Work out the finished part from the listing and answer in its coordinate system (mm). Face numbers are marked on the shaded views. Coordinates: 2 decimals unless noted, no trailing zeros. Order: outer loops, then holes, each group sorted by start corner. A loop starts at its lowest first (then second) coordinate and runs counter-clockwise, first axis right, second up. Notation, with made-up numbers: (-20, 19.5) -> (4, 19.5) arc R18 cw to (4, 54.5) -> close; hole circle Ø11 at (55, 88). An arc over 180 degrees is marked (long way). Use one line per item in the form item = value.
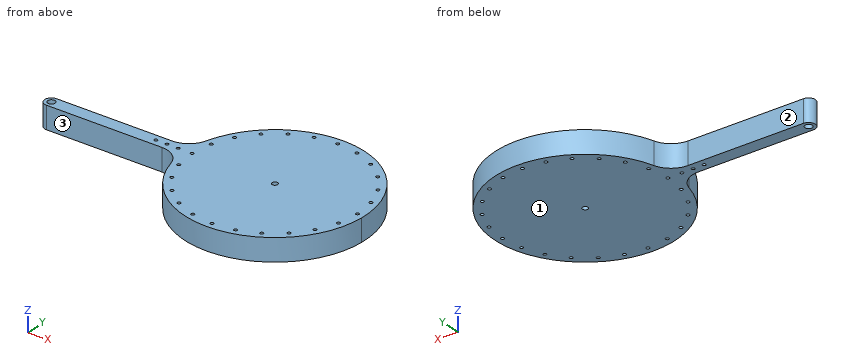
from build123d import *

# Parameters (mm, degrees)
SKETCH1_R           = 1.45
SKETCH1_R_2         = 1.450000001
SKETCH1_R_3         = 3.250000001
SKETCH1_R_4         = 2.5
BOSS_EXTRUDE2_DEPTH = 20


with BuildPart() as part:
    # Sketch1 → Boss-Extrude2 (new body)
    with BuildSketch(Plane.XY):
        with BuildLine():
            Line((-155.352886895, 10.211716756), (-51.913748531, 10.211716756))
            ThreePointArc((-51.913748531, 10.211716756), (-39.74822347, 6.086224622), (-32.601576204, -4.588283244))
            ThreePointArc((-32.601576204, -4.588283244), (53.610301025, -63.284580406), (124.587919611, 13.13479368))
            ThreePointArc((124.587919611, 13.13479368), (56.661218885, 95.304455124), (-32.601576204, 37.011716756))
            ThreePointArc((-32.601576204, 37.011716756), (-39.74822347, 26.33720889), (-51.913748531, 22.211716756))
            Line((-51.913748531, 22.211716756), (-155.352886895, 22.211716756))
            ThreePointArc((-155.352886895, 22.211716756), (-161.352886895, 16.211716756), (-155.352886895, 10.211716756))
        make_face()
        with Locations((-19.438766773, -20.788283244)):
            Circle(SKETCH1_R, mode=Mode.SUBTRACT)
        with Locations((-26.831398039, -2.940892579)):
            Circle(SKETCH1_R_2, mode=Mode.SUBTRACT)
        with Locations((-155.352886895, 16.211716756)):
            Circle(SKETCH1_R_3, mode=Mode.SUBTRACT)
        with Locations((-26.831398039, 35.364326096)):
            Circle(SKETCH1_R_2, mode=Mode.SUBTRACT)
        with Locations((-19.438766774, 53.211716759)):
            Circle(SKETCH1_R_2, mode=Mode.SUBTRACT)
        with Locations((-29.352886893, 16.211716758)):
            Circle(SKETCH1_R_2, mode=Mode.SUBTRACT)
        with Locations((-51.913748531, 16.211716758)):
            Circle(SKETCH1_R, mode=Mode.SUBTRACT)
        with Locations((-41.913748531, 16.211716758)):
            Circle(SKETCH1_R, mode=Mode.SUBTRACT)
        with Locations((-61.913748531, 16.211716758)):
            Circle(SKETCH1_R, mode=Mode.SUBTRACT)
        with Locations((116.125624253, -2.940892579)):
            Circle(SKETCH1_R_2, mode=Mode.SUBTRACT)
        with Locations((108.732992988, -20.788283242)):
            Circle(SKETCH1_R_2, mode=Mode.SUBTRACT)
        with Locations((96.973014915, -36.114185049)):
            Circle(SKETCH1_R_2, mode=Mode.SUBTRACT)
        with Locations((81.647113106, -47.874163121)):
            Circle(SKETCH1_R_2, mode=Mode.SUBTRACT)
        with Locations((63.799722443, -55.266794386)):
            Circle(SKETCH1_R_2, mode=Mode.SUBTRACT)
        with Locations((44.647113106, -57.788283242)):
            Circle(SKETCH1_R_2, mode=Mode.SUBTRACT)
        with Locations((25.494503768, -55.266794386)):
            Circle(SKETCH1_R_2, mode=Mode.SUBTRACT)
        with Locations((7.647113108, -47.874163121)):
            Circle(SKETCH1_R_2, mode=Mode.SUBTRACT)
        with Locations((-7.678788702, -36.114185049)):
            Circle(SKETCH1_R_2, mode=Mode.SUBTRACT)
        with Locations((44.647113106, 16.211716756)):
            Circle(SKETCH1_R_4, mode=Mode.SUBTRACT)
        with Locations((-7.678788702, 68.537618566)):
            Circle(SKETCH1_R_2, mode=Mode.SUBTRACT)
        with Locations((7.647113108, 80.297596638)):
            Circle(SKETCH1_R_2, mode=Mode.SUBTRACT)
        with Locations((25.494503768, 87.690227903)):
            Circle(SKETCH1_R_2, mode=Mode.SUBTRACT)
        with Locations((44.647113106, 90.211716759)):
            Circle(SKETCH1_R_2, mode=Mode.SUBTRACT)
        with Locations((63.799722443, 87.690227903)):
            Circle(SKETCH1_R_2, mode=Mode.SUBTRACT)
        with Locations((81.647113106, 80.297596638)):
            Circle(SKETCH1_R_2, mode=Mode.SUBTRACT)
        with Locations((96.973014915, 68.537618566)):
            Circle(SKETCH1_R_2, mode=Mode.SUBTRACT)
        with Locations((108.732992988, 53.211716759)):
            Circle(SKETCH1_R_2, mode=Mode.SUBTRACT)
        with Locations((116.125624253, 35.364326096)):
            Circle(SKETCH1_R_2, mode=Mode.SUBTRACT)
        with Locations((118.647113104, 16.211716758)):
            Circle(SKETCH1_R_2, mode=Mode.SUBTRACT)
    extrude(amount=BOSS_EXTRUDE2_DEPTH)


solid = part.part
(1) Each of these flat-tipped pins is pushed along its axis until it touches: P1, Ø1, axis at x = -114, z = 7, coming from the +Y side; P2, Ø5, axis at x = -61.5, z = 9.5, coming from the -Y side; P3, Ø1.5, axis at y = -10, z = 13.5, coming from the -X side. Where does it stop, or does it pass through?
Data:
P1 = 22.21
P2 = 10.21
P3 = -31.19
(2) Section B-B on z = 14.5 is taken. Count the separate pieces of the cut face and the enclosed holes in it, plus the area to 3 significant figures.
Data:
separate_pieces = 1
enclosed_holes = 29
area = 21,500 mm²
(3) Section A-A on x = -114.5 is taken. Write down the section's boundary in (y, z), plus the area to 3 significant figures.
Data:
outline = (10.21, 0) -> (22.21, 0) -> (22.21, 20) -> (10.21, 20) -> close
area = 240 mm²
(4) Straight lines are drawn through the part: line 1 along Y through (x, z) = (-27, 6.75); line 2 along X through (y, z) = (-48.5, 10.25); line 3 along X through (y, z) = (54.5, 13). For each, find the intervals that lie inside material, in ascending order.
Data:
line_1 = -19.38 to -4.38, -1.5 to 33.92, 36.8 to 51.8
line_2 = -2.39 to 6.34, 8.96 to 80.34, 82.96 to 91.68
line_3 = -25.6 to -20.1, -18.77 to 108.07, 109.4 to 114.89
(5) Section C-C on y = -30.5 is taken. Write down the section's boundary in (x, z), plus the area to 3 significant figures.
Data:
outline = (-20.3, 0) -> (109.59, 0) -> (109.59, 20) -> (-20.3, 20) -> close
area = 2,600 mm²
(6) The mould has two halves that part along Y. Classify the marked faces 1, 2 and 3: released by +Y, released by -Y, zero draft, split by the parting line, or undercut.
Data:
face_1 = zero draft
face_2 = released by +Y
face_3 = released by -Y
